Can you work these out from the model? Positions are in its coordinate system, mm. Face numbers are marked on the shaded views. Round coordinates to 2 decimals unless told otherwise and drop trailing zeros. Write each loop counter-clockwise with the first axis right and the second up, starting at its lowest first coordinate (ties: lowest second). Pieces come first, ordered by that corner, then holes. Notation, with made-up numbers: (22.5, -7) - (57.5, -7) arc R18 cw to (57.5, 25) - close; hole circle Ø3 at (54, 52). An arc over 180 degrees is marked (long way). One line per item, written item: value. Start each with the question number.
(1) I want a section at B-B on x = 5. List the corners of the cut face in (y, z) for me.
(2) I'm going to push flat-ended pins straight in: pin 1 Ø2 at (x, z) = (-0.5, 7.5) entering from +Y; pin 2 Ø2 at (y, z) = (10.5, 3.5) entering from +X (3 decimals); pin 3 Ø1.3 at (x, y) = (12.5, 11) entering from +Z; pin 4 Ø3 at (x, z) = (16.5, 7) entering from +Y. Where does each tip first touch, or does it pass through?
(3) If I drill on L1, parallel to Y at x = 7.5, z = 3.75; L2, parallel to Z at x = -21, y = -13; L3, parallel to Z at x = 18, y = -12, over which ranges is the centre line in solid material (lowest first)? Write a range as from..to.
(4) I want a section at D-D on y = 7. List the corners of the cut face in (x, z) for me, plus the area to 3 significant figures.
(5) Thinking about a two-plate mould opening in Y: for the marked faces 1, 2 and 3, which applies, +Y half, -Y half, draft (parallel to the pull), parting line (faces both ways), or undercut?
(6) I want a section at A-A on z = 4.5. Give the number of separate pieces and of enclosed holes in the cut face, plus the area to 3 significant figures.
from build123d import *

# Parameters (mm, degrees)
SKETCH1_W              = 63.754
SKETCH1_H              = 30.48
BOSS_EXTRUDE1_DEPTH    = 0.889
SKETCH2_W              = 20.574
SKETCH2_H              = 2.54
BOSS_EXTRUDE2_DEPTH    = 4.572
SKETCH3_W              = 0.635
SKETCH3_H              = 0.635
BOSS_EXTRUDE3_DEPTH    = 8.255
FILLET3_R              = 0.127
FILLET4_R              = 0.127
LPATTERN1_COUNT        = 6
LPATTERN1_PITCH        = 2.54
FILLET3_OF_LPATTERN1_R = 0.127
FILLET4_OF_LPATTERN1_R = 0.127
SKETCH4_W              = 15.24
SKETCH4_H              = 2.54
BOSS_EXTRUDE4_DEPTH    = 2.54


with BuildPart() as part:
    # Sketch1 → Boss-Extrude1 (new body, symmetric)
    with BuildSketch(Plane.XY):
        Rectangle(SKETCH1_W, SKETCH1_H)
    extrude(amount=BOSS_EXTRUDE1_DEPTH, both=True)

    # Sketch2 → Boss-Extrude2 (add)
    with BuildSketch(Plane.XY.offset(0.889)):
        with Locations((14.478, 11.1125)):
            Rectangle(SKETCH2_W, SKETCH2_H)
    boss_extrude2 = extrude(amount=BOSS_EXTRUDE2_DEPTH)

    # Mirror1: Boss-Extrude2 across plane
    add(boss_extrude2.mirror(Plane.ZX))

    # Sketch3 → Boss-Extrude3 (add)
    with BuildSketch(Plane.XY.offset(0.889)):
        with Locations((-11.2395, -12.8905)):
            Rectangle(SKETCH3_W, SKETCH3_H)
    boss_extrude3 = extrude(amount=BOSS_EXTRUDE3_DEPTH)

    # Fillet3
    fillet3_edges = [part.edges().sort_by_distance(p)[0] for p in [
        (-10.922, -13.208, 5.0165),
        (-10.922, -12.573, 5.0165),
        (-11.557, -12.573, 5.0165),
        (-11.557, -13.208, 5.0165),
    ]]
    fillet(fillet3_edges, radius=FILLET3_R)

    # Fillet4
    fillet4_edges = [part.edges().sort_by_distance(p)[0] for p in [
        (-10.922, -12.8905, 9.144),
        (-11.2395, -13.208, 9.144),
        (-11.2395, -12.573, 9.144),
        (-11.557, -12.8905, 9.144),
        (-11.519802561, -12.610197439, 9.144),
        (-10.959197439, -12.610197439, 9.144),
        (-11.519802561, -13.170802561, 9.144),
        (-10.959197439, -13.170802561, 9.144),
    ]]
    fillet(fillet4_edges, radius=FILLET4_R)

    # LPattern1: Boss-Extrude3 ×6
    with Locations(*[(i * LPATTERN1_PITCH, 0, 0) for i in range(1, LPATTERN1_COUNT)]):
        add(boss_extrude3)

    # Fillet3 of LPattern1
    fillet3_of_lpattern1_edges = [part.edges().sort_by_distance(p)[0] for p in [
        (-8.382, -13.208, 5.0165),
        (-8.382, -12.573, 5.0165),
        (-9.017, -12.573, 5.0165),
        (-9.017, -13.208, 5.0165),
        (-5.842, -13.208, 5.0165),
        (-5.842, -12.573, 5.0165),
        (-6.477, -12.573, 5.0165),
        (-6.477, -13.208, 5.0165),
        (-3.302, -13.208, 5.0165),
        (-3.302, -12.573, 5.0165),
        (-3.937, -12.573, 5.0165),
        (-3.937, -13.208, 5.0165),
        (-0.762, -13.208, 5.0165),
        (-0.762, -12.573, 5.0165),
        (-1.397, -12.573, 5.0165),
        (-1.397, -13.208, 5.0165),
        (1.778, -13.208, 5.0165),
        (1.778, -12.573, 5.0165),
        (1.143, -12.573, 5.0165),
        (1.143, -13.208, 5.0165),
    ]]
    fillet(fillet3_of_lpattern1_edges, radius=FILLET3_OF_LPATTERN1_R)

    # Fillet4 of LPattern1
    fillet4_of_lpattern1_edges = [part.edges().sort_by_distance(p)[0] for p in [
        (-8.382, -12.8905, 9.144),
        (-8.6995, -13.208, 9.144),
        (-8.6995, -12.573, 9.144),
        (-9.017, -12.8905, 9.144),
        (-8.979802561, -12.610197439, 9.144),
        (-8.419197439, -12.610197439, 9.144),
        (-8.979802561, -13.170802561, 9.144),
        (-8.419197439, -13.170802561, 9.144),
        (-5.842, -12.8905, 9.144),
        (-6.1595, -13.208, 9.144),
        (-6.1595, -12.573, 9.144),
        (-6.477, -12.8905, 9.144),
        (-6.439802561, -12.610197439, 9.144),
        (-5.879197439, -12.610197439, 9.144),
        (-6.439802561, -13.170802561, 9.144),
        (-5.879197439, -13.170802561, 9.144),
        (-3.302, -12.8905, 9.144),
        (-3.6195, -13.208, 9.144),
        (-3.6195, -12.573, 9.144),
        (-3.937, -12.8905, 9.144),
        (-3.899802561, -12.610197439, 9.144),
        (-3.339197439, -12.610197439, 9.144),
        (-3.899802561, -13.170802561, 9.144),
        (-3.339197439, -13.170802561, 9.144),
        (-0.762, -12.8905, 9.144),
        (-1.0795, -13.208, 9.144),
        (-1.0795, -12.573, 9.144),
        (-1.397, -12.8905, 9.144),
        (-1.359802561, -12.610197439, 9.144),
        (-0.799197439, -12.610197439, 9.144),
        (-1.359802561, -13.170802561, 9.144),
        (-0.799197439, -13.170802561, 9.144),
        (1.778, -12.8905, 9.144),
        (1.4605, -13.208, 9.144),
        (1.4605, -12.573, 9.144),
        (1.143, -12.8905, 9.144),
        (1.180197439, -12.610197439, 9.144),
        (1.740802561, -12.610197439, 9.144),
        (1.180197439, -13.170802561, 9.144),
        (1.740802561, -13.170802561, 9.144),
    ]]
    fillet(fillet4_of_lpattern1_edges, radius=FILLET4_OF_LPATTERN1_R)

    # Sketch4 → Boss-Extrude4 (add)
    with BuildSketch(Plane.XY.offset(0.889)):
        with Locations((-4.8895, -12.8905)):
            Rectangle(SKETCH4_W, SKETCH4_H)
    extrude(amount=BOSS_EXTRUDE4_DEPTH)


solid = part.part
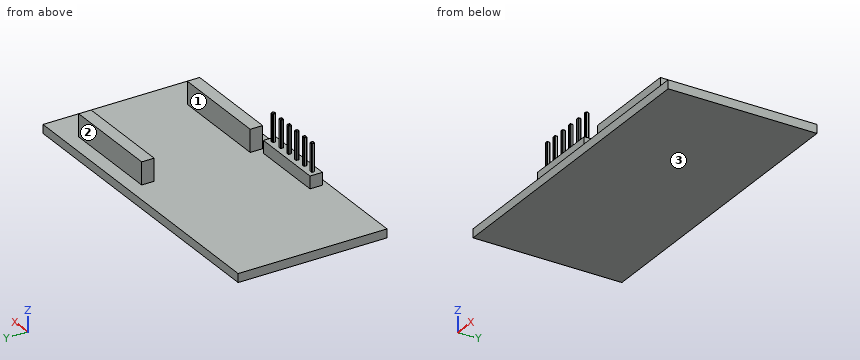
Established:
1. outline: (-15.24, -0.89) - (15.24, -0.89) - (15.24, 0.89) - (12.38, 0.89) - (12.38, 5.46) - (9.84, 5.46) - (9.84, 0.89) - (-9.84, 0.89) - (-9.84, 5.46) - (-12.38, 5.46) - (-12.38, 0.89) - (-15.24, 0.89) - close
2. pin 1: y = -12.57
2. pin 2: x = 24.765
2. pin 3: z = 5.46
2. pin 4: through
3. L1: -12.38..-9.84, 9.84..12.38
3. L2: -0.89..0.89
3. L3: -0.89..5.46
4. outline: (-31.88, -0.89) - (31.88, -0.89) - (31.88, 0.89) - (-31.88, 0.89) - close
4. area: 113 mm2
5. face 1: undercut
5. face 2: +Y half
5. face 3: draft
6. separate pieces: 8
6. enclosed holes: 0
6. area: 107 mm2
